Input: part model. Units: mm. Frame: model coordinates. A direction names the side the tool comes from. Give positions to 0.01 mm unless a question says otherwise; leave off trailing zeros. Loops run counter-clockwise (first coordinate to the right, second up) from the corner with the lowest first, then second, coordinate; pieces in that order, holes last. Notation, with made-up numbers: M 26.5,-14.5 L 80.5,-14.5 A18 cw 80.5,14.5 Z; hole C 12,15.25 d4. An arc over 180 degrees is marked long. Use a Markdown table: item, result. Add a question column.
from build123d import *

# Parameters (mm, degrees)
CUT_EXTRUDE1_DEPTH = 20
SKETCH3_R          = 2.1
CUT_EXTRUDE2_DEPTH = 10


with BuildPart() as part:
    # Sketch1 → Revolve1 (revolve)
    with BuildSketch(Plane(origin=(0, 0, 0), x_dir=(1, 0, 0), z_dir=(0, 1, 0)), mode=Mode.PRIVATE) as revolve1_sk:
        Polygon((26.693713361, 0), (26.693713361, 10.0105), (46.693713361, 10.0105), (46.693713361, 25), (56.693713361, 25), (56.693713361, 0), align=None)
    revolve(revolve1_sk.sketch.rotate(Axis((26.693713361, 0, 0), (1, 0, 0)), 180), axis=Axis((26.693713361, 0, 0), (1, 0, 0)))

    # Sketch2 → Cut-Extrude1 (cut)
    with BuildSketch(Plane.ZY.offset(-26.693713361)):
        with BuildLine():
            ThreePointArc((1.5, 4.769696007), (0, 5), (-1.5, 4.769696007))
            Line((-1.5, 4.769696007), (-1.5, 3.57))
            Line((-1.5, 3.57), (1.5, 3.57))
            Line((1.5, 3.57), (1.5, 4.769696007))
        make_face()
        with BuildLine():
            Line((-1.5, 3.57), (-1.5, 4.769696007))
            ThreePointArc((-1.5, 4.769696007), (-2.958039892, -4.031128874), (5, 0))
            ThreePointArc((5, 0), (4.031128874, 2.958039892), (1.5, 4.769696007))
            Line((1.5, 4.769696007), (1.5, 3.57))
            Line((1.5, 3.57), (-1.5, 3.57))
        make_face()
        with BuildLine():
            Line((1.5, 6.43), (-1.5, 6.43))
            Line((-1.5, 6.43), (-1.5, 4.769696007))
            ThreePointArc((-1.5, 4.769696007), (0, 5), (1.5, 4.769696007))
            Line((1.5, 4.769696007), (1.5, 6.43))
        make_face()
    extrude(amount=-CUT_EXTRUDE1_DEPTH, mode=Mode.SUBTRACT)

    # Sketch3 → Cut-Extrude2 (cut)
    with BuildSketch(Plane(origin=(56.693713361, 0, 0), x_dir=(0, 0, -1), z_dir=(1, 0, 0))):
        with Locations((0, 17.5)):
            Circle(SKETCH3_R)
        with Locations((17.5, 0)):
            Circle(SKETCH3_R)
        with Locations((0, -17.5)):
            Circle(SKETCH3_R)
        with Locations((-17.5, 0)):
            Circle(SKETCH3_R)
    extrude(amount=-CUT_EXTRUDE2_DEPTH, mode=Mode.SUBTRACT)


solid = part.part
1) Section query A-A, the plane z = 0. Return the cut outline in (x, y).
2) Section query D-D, the plane y = -1. Return the cut outline in (x, z).
3) Section query C-C, the plane y = -17.5. Return the cut outline in (x, z).
4) Contact query for flat-ended pins moving along their axis: P1, Ø5, axis at y = 0, z = -17.5, coming from the -X side; P2, Ø11, axis at y = 1.5, z = -1, coming from the -X side; P3, Ø3, axis at x = 49, z = 1, coming from the -Y side; P4, Ø3.5, axis at x = 39.5, z = 0.5, coming from the -Y side. Output: stop coordinate, or through.
5) Ray query, line 1 (Y direction, x = 53.75, z = 0); line 2 (X direction, y = 20, z = 5); line 3 (Z direction, x = 47.75, y = 18). Return the intervals inside material, ascending. Write a range as [from, to].
6) Reachability of faces 1 (the flat face through (37, 6, -1.5)), 2 (the flat face through (56.694, 0, 0)) from +Z, -Z, +X, -X, +Y, -Y: full face, straight path, thin tool, end or side. Return the list, or none.
7) Section query B-B, the plane x = 52.5. Return the cut outline in (y, z).
8) Pull-direction query (Z, two-part tool) for faces 3 (the flat face through (37, 6.43, 0)), 4 (the flat face through (46.694, 11, 0)), 5 (the cylindrical face through (36.83, 8.88, 4.62)); classes: pulls with the +Z half, pulls with the -Z half, needs draft (parallel to the pull), parting line crosses it, or undercut.
Entries:
| question | item | result |
|---|---|---|
| 1 | outline | M 26.69,-10.01 L 46.69,-10.01 L 46.69,-15.4 L 56.69,-15.4 L 56.69,15.4 L 46.69,15.4 L 46.69,10.01 L 26.69,10.01 L 26.69,6.43 L 46.69,6.43 L 46.69,-5 L 26.69,-5 Z; M 46.69,-25 L 56.69,-25 L 56.69,-19.6 L 46.69,-19.6 Z; M 46.69,19.6 L 56.69,19.6 L 56.69,25 L 46.69,25 Z |
| 2 | outline | M 26.69,-9.96 L 46.69,-9.96 L 46.69,-15.65 L 56.69,-15.65 L 56.69,15.65 L 46.69,15.65 L 46.69,9.96 L 26.69,9.96 L 26.69,4.9 L 46.69,4.9 L 46.69,-4.9 L 26.69,-4.9 Z; M 46.69,-24.98 L 56.69,-24.98 L 56.69,-19.35 L 46.69,-19.35 Z; M 46.69,19.35 L 56.69,19.35 L 56.69,24.98 L 46.69,24.98 Z |
| 3 | outline | M 46.69,-17.85 L 56.69,-17.85 L 56.69,-2.1 L 46.69,-2.1 Z; M 46.69,2.1 L 56.69,2.1 L 56.69,17.85 L 46.69,17.85 Z |
| 4 | P1 | stops at x = 46.69 |
| 4 | P2 | stops at x = 26.69 |
| 4 | P3 | stops at y = -25 |
| 4 | P4 | stops at y = -10.01 |
| 5 | line 1 | y = [-25, -19.6], [-15.4, 15.4], [19.6, 25] |
| 5 | line 2 | x = [46.69, 56.69] |
| 5 | line 3 | z = [-17.35, -2.04], [2.04, 17.35] |
| 6 | face 1 | -X |
| 6 | face 2 | +Z, -Z, +X, +Y, -Y |
| 7 | outline | C 0,0 d50; hole C -17.5,0 d4.2; hole C 0,-17.5 d4.2; hole C 0,17.5 d4.2; hole C 17.5,0 d4.2 |
| 8 | face 3 | undercut |
| 8 | face 4 | needs draft |
| 8 | face 5 | parting line crosses it |
